Here's how the part is built. I have some questions about the finished solid (model axes, mm). A direction names the side the tool comes from. Coordinates: 2 decimals unless noted, no trailing zeros. Order: outer loops, then holes, each group sorted by start corner. A loop starts at its lowest first (then second) coordinate and runs counter-clockwise, first axis right, second up.
```python
from build123d import *

# Parameters (mm, degrees)
BOSS_EXTRUDE1_DEPTH     = 57
SKETCH2_R               = 37.5
BOSS_EXTRUDE2_DEPTH     = 2
CUT_EXTRUDE1_DEPTH      = 186.90387301
CUT_EXTRUDE1_DEPTH_BACK = 186.90387301
SKETCH3_W               = 113.978189674
SKETCH3_H               = 54
BODY_MOVE_COPY1_ANGLE   = 90


with BuildPart() as part:
    # Sketch1 → Boss-Extrude1 (new, symmetric)
    with BuildSketch(Plane.XY):
        with BuildLine():
            Line((-165, -58.5), (-165, 58.5))
            Line((-165, 58.5), (2.552640416, 49.934797756))
            ThreePointArc((2.552640416, 49.934797756), (50, 0), (2.552640416, -49.934797756))
            Line((2.552640416, -49.934797756), (-165, -58.5))
        make_face()
    extrude(amount=BOSS_EXTRUDE1_DEPTH, both=True)

    # Sketch2 → Boss-Extrude2 (add)
    with BuildSketch(Plane.ZY.offset(165)):
        Circle(SKETCH2_R)
    extrude(amount=BOSS_EXTRUDE2_DEPTH)

    # Sketch3 → Cut-Extrude1 (cut, two sides: drawn at the far end of the back side and taken through both)
    with BuildSketch(Plane(origin=(0, 0, 0), x_dir=(1, 0, 0), z_dir=(0, 1, 0)).offset(-CUT_EXTRUDE1_DEPTH_BACK)):
        with Locations((-3.010905163, 0)):
            Rectangle(SKETCH3_W, SKETCH3_H)
    extrude(amount=CUT_EXTRUDE1_DEPTH + CUT_EXTRUDE1_DEPTH_BACK, mode=Mode.SUBTRACT)


with BuildPart() as part_1:
    # Body-Move/Copy1: moved
    add(part.part.rotate(Axis((0, 0, 0), (0, 0, 1)), BODY_MOVE_COPY1_ANGLE))


solid = part_1.part
```
Q1. I need wall thicknesses on L1, parallel to Z at x = 32, y = -18; L2, parallel to Y at x = 16, z = 1; L3, parallel to Y at x = -3, z = -37.5. Which ranges of each line are inside material? Lowest first, please.
Q2. If we section it at C-C on x = 0: Write out the boundary of the cut face in (y, z).
Q3. If we section it at B-B on z = 0: Write out the boundary of the cut face in (x, y).
Q4. Will these pins go through, and if not, where does the flat tip stop? pin 1 (4 mm diameter, centred on x = 30, z = 8.5, fed in from +Y); pin 2 (10 mm diameter, centred on y = -87.5, z = 36, fed in from +X); pin 3 (12 mm diameter, centred on y = -15.5, z = -35.5, fed in from -X).
Q5. If we section it at D-D on x = -33: Write out the boundary of the cut face in (y, z), then the cut area to 3 significant figures.
Q6. For faces 1 (the flat face through (1, -165, 39)), 2 (the flat face through (-55.23, -101.01, 0.8)), 3 (the flat face through (1, -6, -27)), which set-ups out of +Z, -Z, +X, -X, +Y, -Y let a thin tool reach every point of the face, with its end or its side?
Q7. If we section it at A-A on y = 0: Write out the boundary of the cut face in (x, z), then the cut area to 3 significant figures.
Reply:
1. L1: z = -57 to -27, 27 to 57
1. L2: y = -167 to -60
1. L3: y = -165 to 49.91
2. outline: (-167, -37.5) - (-165, -37.5) - (-165, -57) - (50, -57) - (50, -27) - (-60, -27) - (-60, 27) - (50, 27) - (50, 57) - (-165, 57) - (-165, 37.5) - (-167, 37.5) - close
3. outline: (-58.5, -165) - (-37.5, -165) - (-37.5, -167) - (37.5, -167) - (37.5, -165) - (58.5, -165) - (53.13, -60) - (-53.13, -60) - close
4. pin 1: stops at y = -60
4. pin 2: stops at x = 54.79
4. pin 3: stops at x = -51.16
5. outline: (-167, -17.81) - (-165, -17.81) - (-165, -57) - (37.56, -57) - (37.56, -27) - (-60, -27) - (-60, 27) - (37.56, 27) - (37.56, 57) - (-165, 57) - (-165, 17.81) - (-167, 17.81) - close
5. area: 17,900 mm2
6. face 1: -Y
6. face 2: +Z, -Z, -X, +Y
6. face 3: +X, -X, +Y
7. outline: (-50.07, -57) - (50.07, -57) - (50.07, -27) - (-50.07, -27) - close; (-50.07, 27) - (50.07, 27) - (50.07, 57) - (-50.07, 57) - close
7. area: 6,010 mm2
